Could you check a few things on this model? Use its own coordinates, in mm. Face numbers are marked on the shaded views. Round coordinates to 2 decimals unless told otherwise and drop trailing zeros. Loops run counter-clockwise (first coordinate to the right, second up) from the corner with the lowest first, then second, coordinate; pieces in that order, holes last. Notation, with made-up numbers: M -34,40 L -21,40 A24 cw -21,68 Z; hole C -14,63.5 d11. An arc over 180 degrees is marked long. Answer in a Markdown table with one row per item.
```python
from build123d import *

# Parameters (mm, degrees)
SKETCH_1_R          = 1
EXTRUDE_1_DEPTH     = 2
SKETCH_2_W          = 1.3
SKETCH_2_H          = 56
EXTRUDE_2_DEPTH     = 3
SKETCH_3_W          = 10
SKETCH_3_H          = 11
SKETCH_3_W_2        = 20
SKETCH_3_H_2        = 14
CUT_EXTRUDE_1_DEPTH = 1.2
SKETCH_4_W          = 1.3
SKETCH_4_H          = 3.5
CUT_EXTRUDE_2_DEPTH = 1


with BuildPart() as part:
    # 草图1 → 凸台-拉伸1 (new body)
    with BuildSketch(Plane.XY):
        Polygon((18.5, 15), (-18.5, 15), (-18.5, 17), (-17, 18.5), (-17, 28), (-33, 28), (-33, -28), (-18.5, -28), (-18.5, -17), (-18.5, -15), (18.5, -15), (18.5, -17), (17, -18.5), (17, -28), (33, -28), (33, 28), (17, 28), (17, 18.5), (18.5, 17), align=None)
        with Locations((19, -20)):
            Circle(SKETCH_1_R, mode=Mode.SUBTRACT)
        with Locations((-19, 20)):
            Circle(SKETCH_1_R, mode=Mode.SUBTRACT)
        with Locations((19, 20)):
            Circle(SKETCH_1_R, mode=Mode.SUBTRACT)
    extrude(amount=EXTRUDE_1_DEPTH)

    # 草图2 → 凸台-拉伸2 (add)
    with BuildSketch(Plane.XY.offset(2)):
        with Locations((-32.35, 0)):
            Rectangle(SKETCH_2_W, SKETCH_2_H)
        with Locations((32.35, 0)):
            Rectangle(SKETCH_2_W, SKETCH_2_H)
        with Locations((-29.35, 0)):
            Rectangle(SKETCH_2_W, SKETCH_2_H)
        with Locations((-26.35, 0)):
            Rectangle(SKETCH_2_W, SKETCH_2_H)
        with Locations((-23.35, 0)):
            Rectangle(SKETCH_2_W, SKETCH_2_H)
        with Locations((29.35, 0)):
            Rectangle(SKETCH_2_W, SKETCH_2_H)
        with Locations((26.35, 0)):
            Rectangle(SKETCH_2_W, SKETCH_2_H)
        with Locations((23.35, 0)):
            Rectangle(SKETCH_2_W, SKETCH_2_H)
    extrude(amount=EXTRUDE_2_DEPTH)

    # 草图3 → 切除-拉伸1 (cut)
    with BuildSketch(Plane(origin=(0, 0, 0), x_dir=(-1, 0, 0), z_dir=(0, 0, -1))):
        Polygon((-15, -3), (-15, 15), (-18.5, 15), (-33, 15), (-33, -3), (-23, -3), align=None)
        with Locations((-28, -8.5)):
            Rectangle(SKETCH_3_W, SKETCH_3_H)
        with Locations((0, 4)):
            Rectangle(SKETCH_3_W_2, SKETCH_3_H_2)
    extrude(amount=-CUT_EXTRUDE_1_DEPTH, mode=Mode.SUBTRACT)

    # 草图4 → 切除-拉伸2 (cut)
    with BuildSketch(Plane.XY.offset(5)):
        with Locations((32.35, -10.25)):
            Rectangle(SKETCH_4_W, SKETCH_4_H)
    extrude(amount=-CUT_EXTRUDE_2_DEPTH, mode=Mode.SUBTRACT)


solid = part.part
```
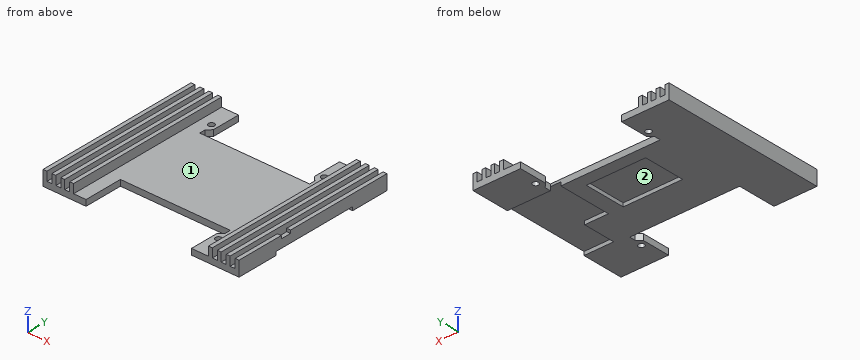
1) Will these pins go through, and if not, where does the flat tip stop? P1, Ø1.5, axis at x = 12, z = 1.5, coming from the +Y side; P2, Ø1.4, axis at x = 32.5, y = -10.5, coming from the +Z side; P3, Ø1, axis at x = 3, z = 0.5, coming from the -Y side.
Computed:
| item | result |
|---|---|
| P1 | stops at y = 15 |
| P2 | stops at z = 4 |
| P3 | stops at y = -15 |
2) I need wall thicknesses on line 1 (Y direction, x = 19, z = 1.5); line 2 (Y direction, x = 19, z = 0.5); line 3 (X direction, y = 25, z = 0.45). Which ranges of each line are inside material? Lowest first, please.
Computed:
| item | result |
|---|---|
| line 1 | y = -28 to -21, -19 to 19, 21 to 28 |
| line 2 | y = -28 to -21, -19 to -3, 15 to 19, 21 to 28 |
| line 3 | x = -33 to -17, 17 to 33 |
3) I want a section at A-A, the plane x = 25. Please give me the cut outline in (y, z), plus the area to 3 significant figures.
Computed:
| item | result |
|---|---|
| outline | M -28,0 L -14,0 L -14,1.2 L 15,1.2 L 15,0 L 28,0 L 28,2 L -28,2 Z |
| area | 77.2 mm² |
4) I want a section at B-B, the plane y = -20. State how many separate pieces and enclosed holes the cut face has, plus the area to 3 significant figures.
Computed:
| item | result |
|---|---|
| separate pieces | 3 |
| enclosed holes | 0 |
| area | 88.2 mm² |
5) If we mould it in two halves opening along Y, with no side actions, what happens to the marked faces 1 and 2? For each: released by +Y, released by -Y, zero draft, split by the parting line, or undercut.
Computed:
| item | result |
|---|---|
| face 1 | zero draft |
| face 2 | undercut |
6) I want a section at D-D, the plane x = -2. Please give me the cut outline in (y, z), plus the area to 3 significant figures.
Computed:
| item | result |
|---|---|
| outline | M -15,0 L -3,0 L -3,1.2 L 11,1.2 L 11,0 L 15,0 L 15,2 L -15,2 Z |
| area | 43.2 mm² |
